The listing builds one solid part. Answer for the finished solid, in the listing's coordinates (mm). Coordinates: 2 decimals unless noted, no trailing zeros. Order: outer loops, then holes, each group sorted by start corner. A loop starts at its lowest first (then second) coordinate and runs counter-clockwise, first axis right, second up. Notation, with made-up numbers: (-27.5, 35.25) -> (-4.5, 35.25) arc R29 cw to (-4.5, 61.25) -> close; hole circle Ø2 at (-10.5, -2). An arc over 180 degrees is marked (long way). Write item = value, one per line.
Autodesk Inventor part; units mm, degrees
ref_plane "YZ Plane" through (0, 0, 0) normal (1, 0, 0) x (0, 1, 0)
ref_plane "XZ Plane" through (0, 0, 0) normal (0, 1, 0) x (-1, 0, 0)
ref_plane "XY Plane" through (0, 0, 0) normal (0, 0, 1) x (1, 0, 0)
ref_plane "Work Plane1" through (816103.6043, 395739.5889, 5886.7052) normal (0, 0, 1) x (1, 0, 0)
sketch "Sketch1" plane through (816103.6043, 395739.5889, 5886.7052) normal (0, 0, 1) x (1, 0, 0)
  line L0 (-6, 7) -> (-16, 7)
  line L1 (-16, 7) -> (-16, -5)
  line L2 (-16, -5) -> (-6, -5)
  line L3 (-6, -5) -> (-6, 7)
  line L4 (-144.5049, 7) -> (-134.5049, 7)
  line L5 (-134.5049, 7) -> (-134.5049, -5)
  line L6 (-134.5049, -5) -> (-144.5049, -5)
  line L7 (-144.5049, -5) -> (-144.5049, 7)
  point P0 (-816103.6043, -395739.5889)
  dimension "d0" = 10
  dimension "d1" = 12
  dimension "d2" = 10
  dimension "d3" = 12
extrude "Extrusion1" add sketch "Sketch1" against normal blind 450
sketch "Sketch2" plane through (815969.0994, 395734.5889, 5886.7052) normal (1, 0, 0) x (0, 0, -1)
  circle A0 centre (6, 6) radius 2.25
  point P0 (5886.7052, -395734.5889)
  dimension "d6" = 4.5
extrude "Extrusion2" add sketch "Sketch2" along normal blind 130
properties part number "antebrazo"
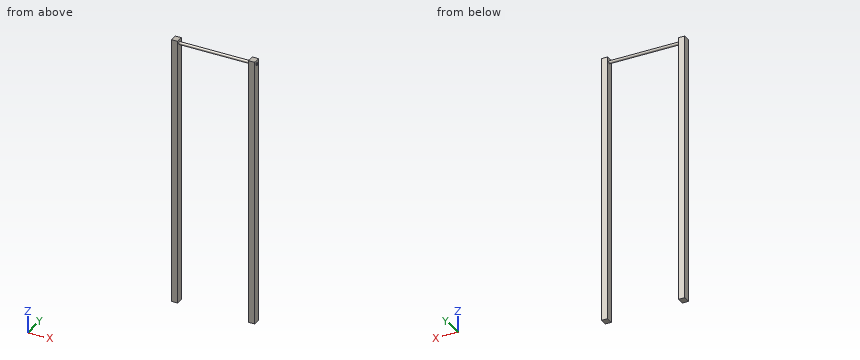
Q1. Section A-A, the plane z = 5494 is taken. Give the vertices of the cut face in (x, y).
The answers:
outline = (815959.1, 395734.59) -> (815969.1, 395734.59) -> (815969.1, 395746.59) -> (815959.1, 395746.59) -> close; (816087.6, 395734.59) -> (816097.6, 395734.59) -> (816097.6, 395746.59) -> (816087.6, 395746.59) -> close
Q2. Find the intervals of material crossed by line 1 along X through (y, z) = (395745, 5764); line 2 along Z through (x, y) = (815992.5, 395740.25); line 3 along Z through (x, y) = (816087.5, 395742.25), in increasing order.
The answers:
line_1 = 815959.1 to 815969.1, 816087.6 to 816097.6
line_2 = 5878.48 to 5882.93
line_3 = 5879.19 to 5882.22
Q3. Section C-C, the plane x = 816043 is taken. Give the vertices of the cut face in (y, z), plus the area to 3 significant figures.
The answers:
outline = circle Ø4.5 at (395740.59, 5880.71)
area = 15.9 mm2
Q4. This flat-tipped pin is pushed along its axis until it touches: pin 1 Ø2 at (y, z) = (395739.5, 5702) entering from +X. Where does it stop, or does it pass through?
The answers:
pin_1 = 816097.6
Q5. Section B-B, the plane y = 395736.5 is taken. Give the vertices of the cut face in (x, z), plus the area to 3 significant figures.
The answers:
outline = (815959.1, 5436.71) -> (815969.1, 5436.71) -> (815969.1, 5886.71) -> (815959.1, 5886.71) -> close; (816087.6, 5436.71) -> (816097.6, 5436.71) -> (816097.6, 5886.71) -> (816087.6, 5886.71) -> close
area = 9,000 mm2
